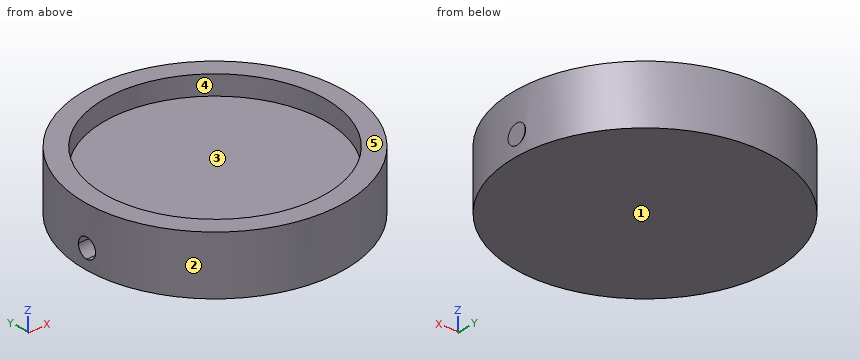
```python
from build123d import *

# Parameters (mm, degrees)
F0_R     = 33.5
F0_R_2   = 28.5
F1_DEPTH = 15
F2_DEPTH = 10
F4_DEPTH = 35
F5_DEPTH = 33.5
F6_DEPTH = 10


with BuildPart() as f1:
    # F0 (on Top) → F1 (new body)
    with BuildSketch(Plane.XY):
        Circle(F0_R)
        Circle(F0_R_2, mode=Mode.SUBTRACT)
    extrude(amount=F1_DEPTH)

    # F0 (on Top) → F2 (join)
    with BuildSketch(Plane.XY):
        Circle(F0_R_2)
    extrude(amount=F2_DEPTH)

    # F3 (on Right) → F4 (cut, symmetric)
    with BuildSketch(Plane.YZ):
        with BuildLine():
            ThreePointArc((0, 2.5), (1.767767, 3.232233), (2.5, 5))
            ThreePointArc((2.5, 5), (-1.767767, 6.767767), (0, 2.5))
        make_face()
    extrude(amount=F4_DEPTH, both=True, mode=Mode.SUBTRACT)

    # F3 (on Right) → F5 (join)
    with BuildSketch(Plane.YZ):
        with BuildLine():
            ThreePointArc((0, 2.5), (1.767767, 3.232233), (2.5, 5))
            ThreePointArc((2.5, 5), (-1.767767, 6.767767), (0, 2.5))
        make_face()
    extrude(amount=F5_DEPTH)

    # F3 (on Right) → F6 (cut)
    with BuildSketch(Plane.YZ):
        with BuildLine():
            ThreePointArc((0, 2.5), (1.767767, 3.232233), (2.5, 5))
            ThreePointArc((2.5, 5), (-1.767767, 6.767767), (0, 2.5))
        make_face()
    extrude(amount=F6_DEPTH, mode=Mode.SUBTRACT)


solid = f1.part
```
Source: CAD feature listing. Evaluate the final solid. Frame: model axes, mm. Face numbers are marked on the shaded views. A direction names the side the tool comes from. Coordinates: 2 decimals unless noted, no trailing zeros. Order: outer loops, then holes, each group sorted by start corner. A loop starts at its lowest first (then second) coordinate and runs counter-clockwise, first axis right, second up. Notation, with made-up numbers: (55, -10) - (89, -10) arc R20 cw to (89, 27) - close; hole circle Ø9 at (14, -2). An arc over 180 degrees is marked (long way). One line per item, written item: value.
1) Cut plane D-D on x = -23. Output: boundary loops of the cut face in (y, z).
Computed values:
outline: (-24.36, 0) - (24.36, 0) - (24.36, 15) - (16.83, 15) - (16.83, 10) - (-16.83, 10) - (-16.83, 15) - (-24.36, 15) - close; hole circle Ø5 at (0, 5)
2) Contact query for flat-ended pins moving along their axis: pin 1 (1 mm diameter, centred on y = -23.5, z = 10.5, fed in from +X); pin 2 (1 mm diameter, centred on y = 20.5, z = 3.5, fed in from +X); pin 3 (5 mm diameter, centred on y = -21.5, z = 7.5, fed in from -X). Output: stop coordinate, or through.
Computed values:
pin 1: stops at x = 24.36
pin 2: stops at x = 26.87
pin 3: stops at x = -27.59
3) Mould query, pull axis X, two halves, no side actions, for the marked faces 1, 2 and 3. Classes: released by +X, released by -X, zero draft, split by the parting line, or undercut.
Computed values:
face 1: zero draft
face 2: split by the parting line
face 3: undercut
4) Cut plane A-A on x = 0. Output: boundary loops of the cut face in (y, z), plus the area to 3 significant figures.
Computed values:
outline: (-33.5, 0) - (33.5, 0) - (33.5, 15) - (28.5, 15) - (28.5, 10) - (-28.5, 10) - (-28.5, 15) - (-33.5, 15) - close; hole circle Ø5 at (0, 5)
area: 700 mm^2
5) Ray query, line 1 (X direction, y = 0.5, z = 14.25); line 2 (Z direction, x = 17.5, y = -11). Return the intervals inside material, ascending. Write a range as [from, to].
Computed values:
line 1: x = [-33.5, -28.5], [28.5, 33.5]
line 2: z = [0, 10]
6) Cut plane C-C on z = 6. Output: boundary loops of the cut face in (x, y), plus the area to 3 significant figures.
Computed values:
outline: (-33.42, -2.29) arc R33.5 ccw to (33.42, -2.29) - (33.5, -2.29) - (33.5, 2.29) - (33.42, 2.29) arc R33.5 ccw to (-33.42, 2.29) - (10, 2.29) - (10, -2.29) - close
area: 3,330 mm^2
7) Cut plane B-B on y = 10. Output: boundary loops of the cut face in (x, z).
Computed values:
outline: (-31.97, 0) - (31.97, 0) - (31.97, 15) - (26.69, 15) - (26.69, 10) - (-26.69, 10) - (-26.69, 15) - (-31.97, 15) - close
8) Reachability of the marked faces 4 and 5 from +Z, -Z, +X, -X, +Y, -Y: full face, straight path, thin tool, end or side. Return the list, or none.
Computed values:
face 4: +Z
face 5: +Z, +X, -X, +Y, -Y
